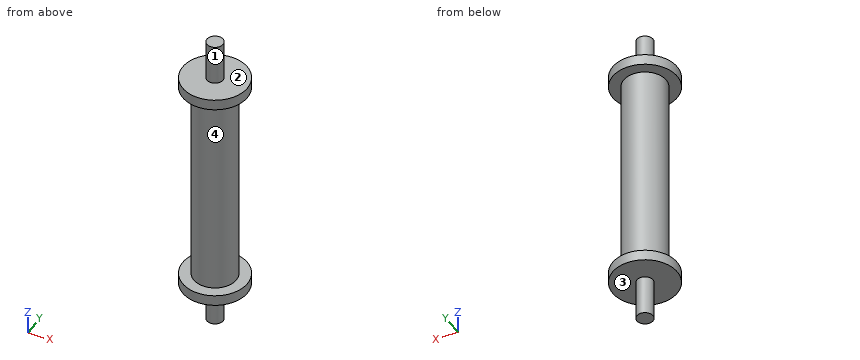
```python
from build123d import *

# Parameters (mm, degrees)
SKETCH1_R           = 3.95
BOSS_EXTRUDE1_DEPTH = 58
SKETCH2_R           = 6
BOSS_EXTRUDE2_DEPTH = 2
BOSS_EXTRUDE3_START = -2
SKETCH3_R           = 6
BOSS_EXTRUDE3_DEPTH = 2
SKETCH4_R           = 4.307153401
SKETCH4_R_2         = 1.5
CUT_EXTRUDE1_DEPTH  = 10
CUT_EXTRUDE2_START  = 10
SKETCH5_R           = 5.180652983
SKETCH5_R_2         = 1.5
CUT_EXTRUDE2_DEPTH  = 10


with BuildPart() as part:
    # Sketch1 → Boss-Extrude1 (new body)
    with BuildSketch(Plane.XY):
        with Locations(Location((0, 0, 0), (0, 0, 180))):
            Circle(SKETCH1_R)
    extrude(amount=BOSS_EXTRUDE1_DEPTH)

    # Sketch2 → Boss-Extrude2 (add)
    with BuildSketch(Plane.XY.offset(50.5)):
        Circle(SKETCH2_R)
    extrude(amount=-BOSS_EXTRUDE2_DEPTH)

    # Sketch3 → Boss-Extrude3 (add)
    with BuildSketch(Plane(origin=(0, 0, 7.5), x_dir=(-1, 0, 0), z_dir=(0, 0, -1)).offset(BOSS_EXTRUDE3_START)):
        with Locations(Location((0, 0, 0), (0, 0, 180))):
            Circle(SKETCH3_R)
    extrude(amount=BOSS_EXTRUDE3_DEPTH)

    # Sketch4 → Cut-Extrude1 (cut)
    with BuildSketch(Plane.XY.offset(50.5)):
        Circle(SKETCH4_R)
        Circle(SKETCH4_R_2, mode=Mode.SUBTRACT)
    extrude(amount=CUT_EXTRUDE1_DEPTH, mode=Mode.SUBTRACT)

    # Sketch5 → Cut-Extrude2 (cut)
    with BuildSketch(Plane(origin=(0, 0, 7.5), x_dir=(-1, 0, 0), z_dir=(0, 0, -1)).offset(CUT_EXTRUDE2_START)):
        Circle(SKETCH5_R)
        with Locations(Location((0, 0, 0), (0, 0, 180))):
            Circle(SKETCH5_R_2, mode=Mode.SUBTRACT)
    extrude(amount=-CUT_EXTRUDE2_DEPTH, mode=Mode.SUBTRACT)


solid = part.part
```
For this review, take the finished solid that the model builds, in its own axes (mm). Face numbers are marked on the shaded views. Round coordinates to 2 decimals unless told otherwise and drop trailing zeros. Write each loop counter-clockwise with the first axis right and the second up, starting at its lowest first coordinate (ties: lowest second). Pieces come first, ordered by that corner, then holes. Notation, with made-up numbers: M -15.5,44.5 L 36.5,44.5 A27 ccw 36.5,79.5 Z; hole C 59.5,-18 d7. An arc over 180 degrees is marked long. One line per item, written item: value. Start each with the question number.
(1) Insertion check: pin 1 (1.5 mm diameter, centred on y = 0.5, z = 47, fed in from +X); pin 2 (4 mm diameter, centred on x = -3.5, z = 22.5, fed in from -Y); pin 3 (5 mm diameter, centred on x = 4, y = 2, fed in from +Z). Each pin has a flat end and moves straight along its axis. Give the tip position at first contact, or say it passes through.
(2) The part is to be moulded in two halves that separate along Z. For the marked faces 1, 2, 3 and 4, say which applies: released by +Z, released by -Z, zero draft, split by the parting line, or undercut.
(3) We need section A-A (x = 0). Give the boundary of the cut face in (y, z).
(4) Wall thickness on line 1 (Z direction, x = 2.5, y = -4); line 2 (Z direction, x = -1.5, y = 0.75); line 3 (Y direction, x = -0.5, z = 26): over which ranges is each line inside the solid? List them lowest first.
(5) We need section D-D (z = 27). Give the boundary of the cut face in (x, y).
(6) We need section C-C (y = -4.5). Give the boundary of the cut face in (x, z), and give its area (3 significant figures).
Result:
1. pin 1: x = 3.95
1. pin 2: y = -3.65
1. pin 3: z = 50.5
2. face 1: zero draft
2. face 2: released by +Z
2. face 3: released by -Z
2. face 4: undercut
3. outline: M -6,7.5 L -1.5,7.5 L -1.5,0 L 1.5,0 L 1.5,7.5 L 6,7.5 L 6,9.5 L 3.95,9.5 L 3.95,48.5 L 6,48.5 L 6,50.5 L 1.5,50.5 L 1.5,58 L -1.5,58 L -1.5,50.5 L -6,50.5 L -6,48.5 L -3.95,48.5 L -3.95,9.5 L -6,9.5 Z
4. line 1: 7.5 to 9.5, 48.5 to 50.5
4. line 2: 7.5 to 50.5
4. line 3: -3.92 to 3.92
5. outline: C 0,0 d7.9
6. outline: M -3.97,7.5 L 3.97,7.5 L 3.97,9.5 L -3.97,9.5 Z; M -3.97,48.5 L 3.97,48.5 L 3.97,50.5 L -3.97,50.5 Z
6. area: 31.7 mm²
